For this review, take the finished solid that the model builds, in its own axes (mm). Give positions to 0.01 mm unless a question says otherwise; leave off trailing zeros. Write each loop counter-clockwise with the first axis right and the second up, starting at its lowest first coordinate (ties: lowest second). Pieces come first, ordered by that corner, then holes.
1) We need section C-C on z = -77. Give the boundary of the cut face in (x, y).
2) We need section D-D on z = 216. Give the boundary of the cut face in (x, y).
3) For P1, Ø12, axis at x = 116.5, z = 144.5, coming from the +Y side; P2, Ø6, axis at x = -46, z = 162.5, coming from the -Y side; P3, Ø4, axis at x = -89, z = 85, coming from the +Y side; P4, Ø6, axis at x = -18, z = -18.5, coming from the +Y side, all flat-tipped, find the tip position at first contact; note any pin that passes through.
4) Wall thickness on line 1 along Z through (x, y) = (-71.5, 46.5); line 2 along X through (y, z) = (133.5, 111.5); line 3 along X through (y, z) = (81, 10.5): over which ranges is each line inside the solid? List them lowest first.
5) We need section A-A on y = 0. Give the boundary of the cut face in (x, z), and give its area (3 significant figures).
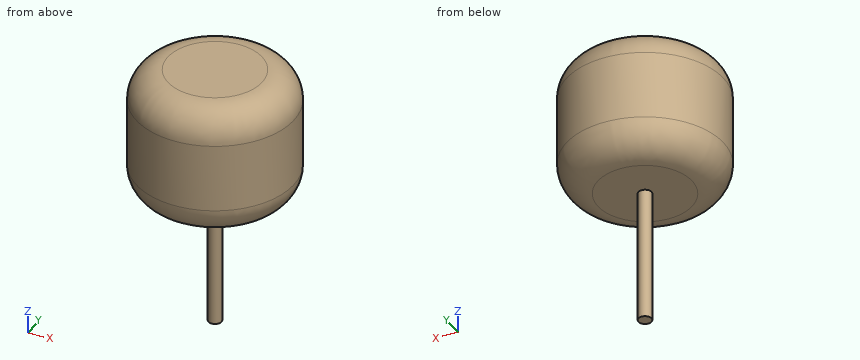
from build123d import *

# Parameters (mm, degrees)
SKETCH2_R           = 150
BOSS_EXTRUDE1_DEPTH = 250
SKETCH3_R           = 12.5
BOSS_EXTRUDE2_DEPTH = 255
FILLET1_R           = 60


with BuildPart() as part:
    # Sketch2 → Boss-Extrude1 (new body)
    with BuildSketch(Plane.XY):
        Circle(SKETCH2_R)
    extrude(amount=BOSS_EXTRUDE1_DEPTH)

    # Sketch3 → Boss-Extrude2 (add)
    with BuildSketch(Plane(origin=(0, 0, 0), x_dir=(-1, 0, 0), z_dir=(0, 0, -1))):
        Circle(SKETCH3_R)
    extrude(amount=BOSS_EXTRUDE2_DEPTH)

    # Fillet1
    fillet1_edges = [part.edges().sort_by_distance(p)[0] for p in [
        (-150, 0, 0),
        (-150, 0, 250),
    ]]
    fillet(fillet1_edges, radius=FILLET1_R)


solid = part.part
Results list:
1. outline: circle Ø25 at (0, 0)
2. outline: circle Ø288.15 at (0, 0)
3. P1: stops at y = 101.44
3. P2: stops at y = -143.7
3. P3: stops at y = 122.19
3. P4: passes through
4. line 1: z = 0 to 250
4. line 2: x = -68.39 to 68.39
4. line 3: x = -93.77 to 93.77
5. outline: (-150, 60) arc R60 ccw to (-90, 0) - (-12.5, 0) - (-12.5, -255) - (12.5, -255) - (12.5, 0) - (90, 0) arc R60 ccw to (150, 60) - (150, 190) arc R60 ccw to (90, 250) - (-90, 250) arc R60 ccw to (-150, 190) - close
5. area: 78,300 mm2
